Here's how the part is built. I have some questions about the finished solid (model axes, mm). A direction names the side the tool comes from. Coordinates: 2 decimals unless noted, no trailing zeros. Write each loop counter-clockwise with the first axis right and the second up, starting at its lowest first coordinate (ties: lowest second). Pieces come first, ordered by that corner, then holes.
(1) Imagine slicing it at B-B, the plane y = -2.25. List the corners of the cut face in (x, z) for me, plus the area to 3 significant figures.
(2) Which directions (+Z, -Z, +X, -X, +Y, -Y) give clear straight access to the entire face, cutting with the end or side of a thin tool? Please do faces 1 (the cylindrical face through (6.19, -1.99, 2.54)), 2 (the flat face through (0, -4, 3)).
(3) For pin 1 Ø3 at (y, z) = (3.5, 1.5) entering from -X; pin 2 Ø1 at (x, z) = (5.5, 2.5) entering from +Y; pin 3 Ø3 at (x, z) = (3, 2) entering from -Y; pin 4 Ø4 at (x, y) = (0, 0) entering from +Z, each with a flat end and sliding along its axis, tell me the tip position at first contact or that it passes through.
(4) Imagine slicing it at A-A, the plane x = 0. List the corners of the cut face in (y, z) for me, plus the area to 3 significant figures.
(5) Please list where these lines run through material, in increasing order: probe 1 along Y at (x, z) = (0, 0.7); probe 2 along Y at (x, z) = (5.25, 0.8).
(6) Thinking about a two-plate mould opening in Y: for faces 3 (the cylindrical face through (-3.804, -5.271, 2.535)), 4 (the cylindrical face through (0, 6.5, 2.5)), 5 (the flat face through (3, 0, 0)), which applies, released by +Y, released by -Y, zero draft, split by the parting line, or undercut?
```python
from build123d import *

# Parameters (mm, degrees)
F0_R     = 7.5
F1_DEPTH = 5
F2_R     = 1
F2_R_2   = 2.5
F3_DEPTH = 25
F5_DEPTH = 3.5


with BuildPart() as f1:
    # F0 (on Top) → F1 (new body)
    with BuildSketch(Plane.XY):
        Circle(F0_R)
    extrude(amount=F1_DEPTH)

    # F2 (on face) → F3 (cut)
    with BuildSketch(Plane.XY.offset(5)):
        with Locations((0, 7.5)):
            Circle(F2_R)
        Circle(F2_R_2)
        with Locations((-2.317627, 7.132924)):
            Circle(F2_R)
        with Locations((-4.408389, 6.067627)):
            Circle(F2_R)
        with Locations((-6.067627, 4.408389)):
            Circle(F2_R)
        with Locations((-7.132924, 2.317627)):
            Circle(F2_R)
        with Locations((-7.5, 0)):
            Circle(F2_R)
        with Locations((-7.132924, -2.317627)):
            Circle(F2_R)
        with Locations((-6.067627, -4.408389)):
            Circle(F2_R)
        with Locations((-4.408389, -6.067627)):
            Circle(F2_R)
        with Locations((-2.317627, -7.132924)):
            Circle(F2_R)
        with Locations((0, -7.5)):
            Circle(F2_R)
        with Locations((2.317627, -7.132924)):
            Circle(F2_R)
        with Locations((4.408389, -6.067627)):
            Circle(F2_R)
        with Locations((6.067627, -4.408389)):
            Circle(F2_R)
        with Locations((7.132924, -2.317627)):
            Circle(F2_R)
        with Locations((7.5, 0)):
            Circle(F2_R)
        with Locations((7.132924, 2.317627)):
            Circle(F2_R)
        with Locations((6.067627, 4.408389)):
            Circle(F2_R)
        with Locations((4.408389, 6.067627)):
            Circle(F2_R)
        with Locations((2.317627, 7.132924)):
            Circle(F2_R)
    extrude(amount=-F3_DEPTH, mode=Mode.SUBTRACT)

    # F4 (on face) → F5 (cut)
    with BuildSketch(Plane.XY.offset(5)):
        Polygon((-2.309401, -4), (2.309401, -4), (4.618802, 0), (2.309401, 4), (-2.309401, 4), (-4.618802, 0), align=None)
    extrude(amount=-F5_DEPTH, mode=Mode.SUBTRACT)


solid = f1.part
```
Recorded:
1. outline: (-6.14, 0) - (-1.09, 0) - (-1.09, 1.5) - (-3.32, 1.5) - (-3.32, 5) - (-6.14, 5) - close; (1.09, 0) - (6.14, 0) - (6.14, 5) - (3.32, 5) - (3.32, 1.5) - (1.09, 1.5) - close
1. area: 34.8 mm2
2. face 1: +Z, -Z
2. face 2: +Z
3. pin 1: stops at x = -6.76
3. pin 2: stops at y = 5.43
3. pin 3: stops at y = -6.76
3. pin 4: passes through
4. outline: (-6.5, 0) - (-2.5, 0) - (-2.5, 1.5) - (-4, 1.5) - (-4, 5) - (-6.5, 5) - close; (2.5, 0) - (6.5, 0) - (6.5, 5) - (4, 5) - (4, 1.5) - (2.5, 1.5) - close
4. area: 29.5 mm2
5. probe 1: y = -6.5 to -2.5, 2.5 to 6.5
5. probe 2: y = -5.36 to -4.98, -3.83 to 3.83, 4.98 to 5.36
6. face 3: undercut
6. face 4: released by +Y
6. face 5: zero draft
